For this review, take the finished solid that the model builds, in its own axes (mm). A direction names the side the tool comes from. Give positions to 0.01 mm unless a question says otherwise; leave off trailing zeros. Loops run counter-clockwise (first coordinate to the right, second up) from the corner with the lowest first, then second, coordinate; pieces in that order, holes last. Notation, with made-up numbers: (-28.5, -6.75) -> (-22.5, -6.75) arc R23 ccw to (-22.5, 30.25) -> close; hole circle Ø8 at (-35, -12.5). An arc over 180 degrees is marked (long way). One line per question, with ' | ' between items. Start each with the question number.
(1) Consider section C-C (z = 64.5). Write out the cut boundary in (x, y).
(2) Insertion check: P1, Ø12, axis at y = 11.5, z = 23, coming from the -X side; P2, Ø8, axis at y = 20, z = 28, coming from the +X side; P3, Ø5, axis at x = -3.5, y = 4.5, coming from the -Z side. Each pin has a flat end and moves straight along its axis. Give the tip position at first contact, or say it passes through.
(3) Consider section B-B (y = 10). Write out the cut boundary in (x, z), and give its area (3 significant figures).
(4) Draft analysis for pull direction X (two halves, no side actions). For faces 1 (the flat face through (0, 21, 102)), 2 (the cylindrical face through (15.58, 2.17, -80.14)), 3 (the cylindrical face through (0.451, 20.495, -82.395)), state which applies: +X half, -X half, draft (parallel to the pull), parting line (faces both ways), or undercut.
(5) Wall thickness on probe 1 along Z at (x, y) = (11.5, 9); probe 2 along X at (y, z) = (9, -4); probe 3 along X at (y, z) = (8.25, -18): over which ranges is each line inside the solid? List them lowest first.
(6) Tool access review of faces 4 (the flat face through (0, 8, 2.5)), 5 (the flat face through (0, 21, -75)), 6 (the flat face through (3, 18, -70)): name each direction out of +Z, -Z, +X, -X, +Y, -Y from which nothing blocks a thin tool from reaching the whole face with its end or side.
(7) Consider section A-A (x = -12). Write out the cut boundary in (y, z).
from build123d import *

# Parameters (mm, degrees)
F3_DEPTH = 2.5
F5_DEPTH = 20
F7_DEPTH = 192.001


with BuildPart() as f1:
    # F0 (on Front) → F1 (revolve)
    with BuildSketch(Plane.XZ):
        Polygon((20.5, 2.5), (0, 2.5), (0, 0), (20.5, 0), (20.5, -70), (18, -70), (18, -90), (20.5, -90), (20.5, -75), (23, -75), (23, 0), (23, 102), (20.5, 102), align=None)
    revolve(axis=Axis((0, 0, 1.25), (0, 0, 1)))

    # F2 (on face) → F3 (cut, through all)
    with BuildSketch(Plane.XY.offset(2.5)):
        with BuildLine():
            Line((0, 12.5), (16.248077, 12.5))
            ThreePointArc((16.248077, 12.5), (9.055385, 18.391574), (0, 20.5))
            Line((0, 20.5), (0, 12.5))
        make_face()
    extrude(amount=-F3_DEPTH, mode=Mode.SUBTRACT)

    # F4 (on face) → F5 (join, through all)
    with BuildSketch(Plane(origin=(0, 0, -90), x_dir=(1, 0, 0), z_dir=(0, 0, -1))):
        with BuildLine():
            ThreePointArc((-17.706597, 3.236729), (-18, 0), (-17.706597, -3.236729))
            ThreePointArc((-17.706597, -3.236729), (-14.75, 0), (-17.706597, 3.236729))
        make_face()
        with BuildLine():
            ThreePointArc((17.706597, -3.236729), (18, 0), (17.706597, 3.236729))
            ThreePointArc((17.706597, 3.236729), (14.75, 0), (17.706597, -3.236729))
        make_face()
    extrude(amount=-F5_DEPTH)

    # F6 (on face) → F7 (cut, through all)
    with BuildSketch(Plane.XY.offset(102)):
        with BuildLine():
            Line((23, 0), (-23, 0))
            ThreePointArc((-23, 0), (0, -23), (23, 0))
        make_face()
    extrude(amount=-F7_DEPTH, mode=Mode.SUBTRACT)


solid = f1.part
A:
1) outline: (-23, 0) -> (-20.5, 0) arc R20.5 cw to (20.5, 0) -> (23, 0) arc R23 ccw to start
2) P1: stops at x = -22.33 | P2: stops at x = 16.52 | P3: stops at z = 0
3) outline: (-20.71, -75) -> (-17.9, -75) -> (-17.9, -90) -> (-14.97, -90) -> (-14.97, -70) -> (-17.9, -70) -> (-17.9, 0) -> (17.9, 0) -> (17.9, -70) -> (14.97, -70) -> (14.97, -90) -> (17.9, -90) -> (17.9, -75) -> (20.71, -75) -> (20.71, 102) -> (17.9, 102) -> (17.9, 2.5) -> (-17.9, 2.5) -> (-17.9, 102) -> (-20.71, 102) -> close | area: 1,200 mm^2
4) face 1: draft | face 2: undercut | face 3: parting line
5) probe 1: z = 0 to 2.5 | probe 2: x = -21.17 to -18.42, 18.42 to 21.17 | probe 3: x = -21.47 to -18.77, 18.77 to 21.47
6) face 4: +Z, -Y | face 5: -Z, +Y | face 6: -Y
7) outline: (0, 0) -> (16.62, 0) -> (16.62, -70) -> (13.42, -70) -> (13.42, -90) -> (16.62, -90) -> (16.62, -75) -> (19.62, -75) -> (19.62, 102) -> (16.62, 102) -> (16.62, 2.5) -> (0, 2.5) -> close
